```python
from build123d import *

# Parameters (mm, degrees)
SKETCH1_R           = 1.6
BOSS_EXTRUDE1_DEPTH = 7.5
SKETCH2_R           = 17.2
BOSS_EXTRUDE2_DEPTH = 7.5


with BuildPart() as part:
    # Sketch1 → Boss-Extrude1 (new body)
    with BuildSketch(Plane(origin=(0, 0, 0), x_dir=(1, 0, 0), z_dir=(0, 1, 0))):
        with BuildLine():
            Line((-5, 43.966606646), (-5, 44.520107817))
            ThreePointArc((-5, 44.520107817), (0, 44.8), (5, 44.520107817))
            Line((5, 44.520107817), (5, 43.966606646))
            ThreePointArc((5, 43.966606646), (31.289475068, 31.289475068), (43.966606646, 5))
            Line((43.966606646, 5), (44.520107817, 5))
            ThreePointArc((44.520107817, 5), (44.8, 0), (44.520107817, -5))
            Line((44.520107817, -5), (43.966606646, -5))
            ThreePointArc((43.966606646, -5), (31.289475068, -31.289475068), (5, -43.966606646))
            Line((5, -43.966606646), (5, -44.520107817))
            ThreePointArc((5, -44.520107817), (0, -44.8), (-5, -44.520107817))
            Line((-5, -44.520107817), (-5, -43.966606646))
            ThreePointArc((-5, -43.966606646), (-31.289475068, -31.289475068), (-43.966606646, -5))
            Line((-43.966606646, -5), (-44.520107817, -5))
            ThreePointArc((-44.520107817, -5), (-44.8, 0), (-44.520107817, 5))
            Line((-44.520107817, 5), (-43.966606646, 5))
            ThreePointArc((-43.966606646, 5), (-31.289475068, 31.289475068), (-5, 43.966606646))
        make_face()
        with Locations(Location((36.25, 0, 0), (0, 0, 270))):
            Circle(SKETCH1_R, mode=Mode.SUBTRACT)
        with Locations(Location((25.632620818, -25.632620818, 0), (0, 0, 270))):
            Circle(SKETCH1_R, mode=Mode.SUBTRACT)
        with Locations(Location((0, -36.25, 0), (0, 0, 270))):
            Circle(SKETCH1_R, mode=Mode.SUBTRACT)
        with Locations(Location((-25.632620818, -25.632620818, 0), (0, 0, 270))):
            Circle(SKETCH1_R, mode=Mode.SUBTRACT)
        with Locations(Location((-36.25, 0, 0), (0, 0, 270))):
            Circle(SKETCH1_R, mode=Mode.SUBTRACT)
        with Locations(Location((-25.632620818, 25.632620818, 0), (0, 0, 270))):
            Circle(SKETCH1_R, mode=Mode.SUBTRACT)
        with Locations(Location((0, 36.25, 0), (0, 0, 270))):
            Circle(SKETCH1_R, mode=Mode.SUBTRACT)
        with Locations(Location((25.632620818, 25.632620818, 0), (0, 0, 270))):
            Circle(SKETCH1_R, mode=Mode.SUBTRACT)
        with BuildLine():
            Line((33.430226046, 5), (36.586370413, 5))
            ThreePointArc((36.586370413, 5), (38.127746073, 5.725574218), (38.550739294, 7.375838926))
            ThreePointArc((38.550739294, 7.375838926), (36.262271651, 15.02032472), (32.474994896, 22.043983453))
            ThreePointArc((32.474994896, 22.043983453), (31.008980156, 22.911795444), (29.406004524, 22.334936712))
            Line((29.406004524, 22.334936712), (25.760059877, 18.688992065))
            Line((25.760059877, 18.688992065), (18.688992065, 25.760059877))
            Line((18.688992065, 25.760059877), (22.334936712, 29.406004524))
            ThreePointArc((22.334936712, 29.406004524), (22.911795444, 31.008980156), (22.043983453, 32.474994896))
            ThreePointArc((22.043983453, 32.474994896), (15.02032472, 36.262271651), (7.375838926, 38.550739294))
            ThreePointArc((7.375838926, 38.550739294), (5.725574218, 38.127746073), (5, 36.586370413))
            Line((5, 36.586370413), (5, 33.430226046))
            ThreePointArc((5, 33.430226046), (4.414213562, 32.016012484), (3, 31.430226046))
            Line((3, 31.430226046), (-3, 31.430226046))
            ThreePointArc((-3, 31.430226046), (-4.414213562, 32.016012484), (-5, 33.430226046))
            Line((-5, 33.430226046), (-5, 36.586370413))
            ThreePointArc((-5, 36.586370413), (-5.725574218, 38.127746073), (-7.375838926, 38.550739294))
            ThreePointArc((-7.375838926, 38.550739294), (-15.02032472, 36.262271651), (-22.043983453, 32.474994896))
            ThreePointArc((-22.043983453, 32.474994896), (-22.911795444, 31.008980156), (-22.334936712, 29.406004524))
            Line((-22.334936712, 29.406004524), (-18.688992065, 25.760059877))
            Line((-18.688992065, 25.760059877), (-25.760059877, 18.688992065))
            Line((-25.760059877, 18.688992065), (-29.406004524, 22.334936712))
            ThreePointArc((-29.406004524, 22.334936712), (-31.008980156, 22.911795444), (-32.474994896, 22.043983453))
            ThreePointArc((-32.474994896, 22.043983453), (-36.262271651, 15.02032472), (-38.550739294, 7.375838926))
            ThreePointArc((-38.550739294, 7.375838926), (-38.127746073, 5.725574218), (-36.586370413, 5))
            Line((-36.586370413, 5), (-33.430226046, 5))
            ThreePointArc((-33.430226046, 5), (-32.016012484, 4.414213562), (-31.430226046, 3))
            Line((-31.430226046, 3), (-31.430226046, -3))
            ThreePointArc((-31.430226046, -3), (-32.016012484, -4.414213562), (-33.430226046, -5))
            Line((-33.430226046, -5), (-36.586370413, -5))
            ThreePointArc((-36.586370413, -5), (-38.127746073, -5.725574218), (-38.550739294, -7.375838926))
            ThreePointArc((-38.550739294, -7.375838926), (-36.262271651, -15.02032472), (-32.474994896, -22.043983453))
            ThreePointArc((-32.474994896, -22.043983453), (-31.008980156, -22.911795444), (-29.406004524, -22.334936712))
            Line((-29.406004524, -22.334936712), (-25.760059877, -18.688992065))
            Line((-25.760059877, -18.688992065), (-18.688992065, -25.760059877))
            Line((-18.688992065, -25.760059877), (-22.334936712, -29.406004524))
            ThreePointArc((-22.334936712, -29.406004524), (-22.911795444, -31.008980156), (-22.043983453, -32.474994896))
            ThreePointArc((-22.043983453, -32.474994896), (-15.02032472, -36.262271651), (-7.375838926, -38.550739294))
            ThreePointArc((-7.375838926, -38.550739294), (-5.725574218, -38.127746073), (-5, -36.586370413))
            Line((-5, -36.586370413), (-5, -33.430226046))
            ThreePointArc((-5, -33.430226046), (-4.414213562, -32.016012484), (-3, -31.430226046))
            Line((-3, -31.430226046), (3, -31.430226046))
            ThreePointArc((3, -31.430226046), (4.414213562, -32.016012484), (5, -33.430226046))
            Line((5, -33.430226046), (5, -36.586370413))
            ThreePointArc((5, -36.586370413), (5.725574218, -38.127746073), (7.375838926, -38.550739294))
            ThreePointArc((7.375838926, -38.550739294), (15.02032472, -36.262271651), (22.043983453, -32.474994896))
            ThreePointArc((22.043983453, -32.474994896), (22.911795444, -31.008980156), (22.334936712, -29.406004524))
            Line((22.334936712, -29.406004524), (18.688992065, -25.760059877))
            Line((18.688992065, -25.760059877), (25.760059877, -18.688992065))
            Line((25.760059877, -18.688992065), (29.406004524, -22.334936712))
            ThreePointArc((29.406004524, -22.334936712), (31.008980156, -22.911795444), (32.474994896, -22.043983453))
            ThreePointArc((32.474994896, -22.043983453), (36.262271651, -15.02032472), (38.550739294, -7.375838926))
            ThreePointArc((38.550739294, -7.375838926), (38.127746073, -5.725574218), (36.586370413, -5))
            Line((36.586370413, -5), (33.430226046, -5))
            ThreePointArc((33.430226046, -5), (32.016012484, -4.414213562), (31.430226046, -3))
            Line((31.430226046, -3), (31.430226046, 3))
            ThreePointArc((31.430226046, 3), (32.016012484, 4.414213562), (33.430226046, 5))
        make_face(mode=Mode.SUBTRACT)
    extrude(amount=BOSS_EXTRUDE1_DEPTH)

    # Sketch2 → Boss-Extrude2 (add)
    with BuildSketch(Plane(origin=(0, 7.5, 0), x_dir=(1, 0, 0), z_dir=(0, 1, 0))):
        with BuildLine():
            Line((13.886291501, 22.2), (-13.886291501, 22.2))
            ThreePointArc((-13.886291501, 22.2), (-15.034341798, 22.428361402), (-16.007611845, 23.078679656))
            Line((-16.007611845, 23.078679656), (-18.688992065, 25.760059877))
            Line((-18.688992065, 25.760059877), (-25.760059877, 18.688992065))
            Line((-25.760059877, 18.688992065), (-23.078679656, 16.007611845))
            ThreePointArc((-23.078679656, 16.007611845), (-22.428361402, 15.034341798), (-22.2, 13.886291501))
            Line((-22.2, 13.886291501), (-22.2, -13.886291501))
            ThreePointArc((-22.2, -13.886291501), (-22.428361402, -15.034341798), (-23.078679656, -16.007611845))
            Line((-23.078679656, -16.007611845), (-25.760059877, -18.688992065))
            Line((-25.760059877, -18.688992065), (-18.688992065, -25.760059877))
            Line((-18.688992065, -25.760059877), (-16.007611845, -23.078679656))
            ThreePointArc((-16.007611845, -23.078679656), (-15.034341798, -22.428361402), (-13.886291501, -22.2))
            Line((-13.886291501, -22.2), (13.886291501, -22.2))
            ThreePointArc((13.886291501, -22.2), (15.034341798, -22.428361402), (16.007611845, -23.078679656))
            Line((16.007611845, -23.078679656), (18.688992065, -25.760059877))
            Line((18.688992065, -25.760059877), (25.760059877, -18.688992065))
            Line((25.760059877, -18.688992065), (23.078679656, -16.007611845))
            ThreePointArc((23.078679656, -16.007611845), (22.428361402, -15.034341798), (22.2, -13.886291501))
            Line((22.2, -13.886291501), (22.2, 13.886291501))
            ThreePointArc((22.2, 13.886291501), (22.428361402, 15.034341798), (23.078679656, 16.007611845))
            Line((23.078679656, 16.007611845), (25.760059877, 18.688992065))
            Line((25.760059877, 18.688992065), (18.688992065, 25.760059877))
            Line((18.688992065, 25.760059877), (16.007611845, 23.078679656))
            ThreePointArc((16.007611845, 23.078679656), (15.034341798, 22.428361402), (13.886291501, 22.2))
        make_face()
        with Locations(Location((0, 0, 0), (0, 0, 270))):
            Circle(SKETCH2_R, mode=Mode.SUBTRACT)
    extrude(amount=-BOSS_EXTRUDE2_DEPTH)


solid = part.part
```
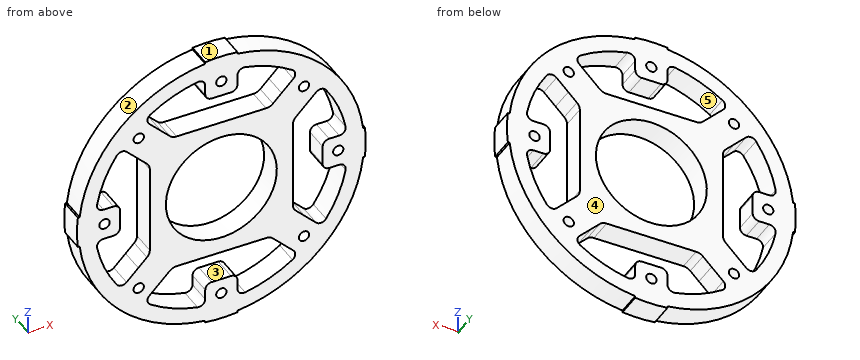
Can you work these out from the model? Positions are in its coordinate system, mm. Face numbers are marked on the shaded views. A direction names the side the tool comes from. Round coordinates to 2 decimals unless told otherwise and drop trailing zeros. Loops run counter-clockwise (first coordinate to the right, second up) from the corner with the lowest first, then second, coordinate; pieces in that order, holes last. Notation, with made-up numbers: M 55.5,15.5 L 67.5,15.5 A19 ccw 67.5,21.5 Z; hole C -34,50 d8. An arc over 180 degrees is marked long. Write item = value, one per line. Start each with the question number.
(1) Which directions (+Z, -Z, +X, -X, +Y, -Y) give clear straight access to the entire face, cutting with the end or side of a thin tool? Please do the marked faces 4 and 5.
(2) Suppose I cut it at C-C on y = 4.75. Give the number of separate pieces and of enclosed holes in the cut face, plus the area to 3 significant figures.
(3) If we mould it in two halves opening along X, with no side actions, what happens to the marked faces 1, 2 and 3? For each: released by +X, released by -X, zero draft, split by the parting line, or undercut.
(4) Suppose I cut it at B-B on x = 0. Write out the boundary of the cut face in (y, z).
(5) I'm going to push flat-ended pins straight in: P1, Ø4, axis at x = 18.5, y = 3.5, coming from the +Z side; P2, Ø2.5, axis at y = 5, z = 34.5, coming from the +X side; P3, Ø3.5, axis at y = 3, z = -35.5, coming from the -X side. Where does each tip first touch, or does it pass through?
(6) I need wall thicknesses on line 1 along X through (y, z) = (5.75, 0); line 2 along Z through (x, y) = (-13.5, 1); line 3 along X through (y, z) = (3, -33). Which ranges of each line are inside material? Lowest first, please.
(7) Suppose I cut it at A-A on z = 0. Write out the boundary of the cut face in (x, y).
Answer block:
q1.face_4 = +Z, -Z, +X, -X, +Y
q1.face_5 = +Y, -Y
q2.separate_pieces = 1
q2.enclosed_holes = 13
q2.area = 3,040 mm²
q3.face_1 = split by the parting line
q3.face_2 = released by -X
q3.face_3 = undercut
q4.outline = M 0,-44.8 L 7.5,-44.8 L 7.5,-37.85 L 0,-37.85 Z; M 0,-34.65 L 7.5,-34.65 L 7.5,-31.43 L 0,-31.43 Z; M 0,-22.2 L 7.5,-22.2 L 7.5,-17.2 L 0,-17.2 Z; M 0,17.2 L 7.5,17.2 L 7.5,22.2 L 0,22.2 Z; M 0,31.43 L 7.5,31.43 L 7.5,34.65 L 0,34.65 Z; M 0,37.85 L 7.5,37.85 L 7.5,44.8 L 0,44.8 Z
q5.P1 = 41.06
q5.P2 = 29.2
q5.P3 = -28.62
q6.line_1 = -44.8 to -37.85, -34.65 to -31.43, -22.2 to -17.2, 17.2 to 22.2, 31.43 to 34.65, 37.85 to 44.8
q6.line_2 = -42.14 to -36.86, -22.2 to -10.66, 10.66 to 22.2, 36.86 to 42.14
q6.line_3 = -29.48 to -21.25, -4.95 to 4.95, 21.25 to 29.48
q7.outline = M -44.8,0 L -37.85,0 L -37.85,7.5 L -44.8,7.5 Z; M -34.65,0 L -31.43,0 L -31.43,7.5 L -34.65,7.5 Z; M -22.2,0 L -17.2,0 L -17.2,7.5 L -22.2,7.5 Z; M 17.2,0 L 22.2,0 L 22.2,7.5 L 17.2,7.5 Z; M 31.43,0 L 34.65,0 L 34.65,7.5 L 31.43,7.5 Z; M 37.85,0 L 44.8,0 L 44.8,7.5 L 37.85,7.5 Z
